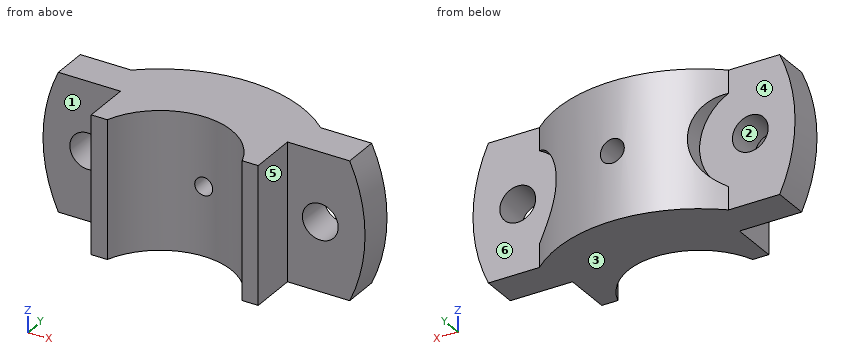
```python
from build123d import *

# Parameters (mm, degrees)
BOSS_EXTRUDE1_DEPTH     = 23
BOSS_EXTRUDE4_START     = 24
BOSS_EXTRUDE4_DEPTH     = 12
SKETCH4_R               = 3
CUT_EXTRUDE1_DEPTH      = 13
CUT_EXTRUDE1_DEPTH_BACK = 29
SKETCH5_R               = 4
CUT_EXTRUDE2_DEPTH      = 16
F_12_0MM_DOWEL_HOLE1_D  = 12
CUT_EXTRUDE3_DEPTH      = 16


with BuildPart() as part:
    # Sketch1 → Boss-Extrude1 (new body, symmetric)
    with BuildSketch(Plane.XY):
        with BuildLine():
            Line((31.749015733, 36), (31.749015733, 24))
            Line((31.749015733, 24), (28, 24))
            Line((28, 24), (28, 8))
            Line((28, 8), (22.627416998, 8))
            ThreePointArc((22.627416998, 8), (0, 24), (-22.627416998, 8))
            Line((-22.627416998, 8), (-28, 8))
            Line((-28, 8), (-28, 24))
            Line((-28, 24), (-31.749015733, 24))
            Line((-31.749015733, 24), (-31.749015733, 36))
            ThreePointArc((-31.749015733, 36), (0, 48), (31.749015733, 36))
        make_face()
    extrude(amount=BOSS_EXTRUDE1_DEPTH, both=True)

    # Sketch3 → Boss-Extrude4 (add)
    with BuildSketch(Plane(origin=(0, 0, 0), x_dir=(1, 0, 0), z_dir=(0, 1, 0)).offset(BOSS_EXTRUDE4_START)):
        with BuildLine():
            Line((31.749015733, -23), (31.749015733, 23))
            Line((31.749015733, 23), (48.856934001, 23))
            ThreePointArc((48.856934001, 23), (54, 0), (48.856934001, -23))
            Line((48.856934001, -23), (31.749015733, -23))
        make_face()
    boss_extrude4 = extrude(amount=BOSS_EXTRUDE4_DEPTH)

    # Mirror2: Boss-Extrude4 across plane
    add(boss_extrude4.mirror(Plane(origin=(0, 0, 0), x_dir=(0, 0, 1), z_dir=(1, 0, 0))))

    # Sketch4 → Cut-Extrude1 (cut, two sides)
    with BuildSketch(Plane(origin=(0, 36, 0), x_dir=(1, 0, 0), z_dir=(0, 1, 0))) as cut_extrude1_sk:
        Circle(SKETCH4_R)
    extrude(amount=CUT_EXTRUDE1_DEPTH, mode=Mode.SUBTRACT)
    extrude(cut_extrude1_sk.sketch, amount=-CUT_EXTRUDE1_DEPTH_BACK, mode=Mode.SUBTRACT)

    # Sketch5 → Cut-Extrude2 (cut)
    with BuildSketch(Plane(origin=(0, 48, 0), x_dir=(1, 0, 0), z_dir=(0, 1, 0))):
        Circle(SKETCH5_R)
    extrude(amount=-CUT_EXTRUDE2_DEPTH, mode=Mode.SUBTRACT)

    # Ø12.0mm Dowel Hole1 (through all)
    with Locations(Plane(origin=(0, 36, 0), x_dir=(1, 0, 0), z_dir=(0, 1, 0))):
        with Locations((-39, 0), (39, 0)):
            Hole(F_12_0MM_DOWEL_HOLE1_D / 2)

    # Sketch8 → Cut-Extrude3 (cut)
    with BuildSketch(Plane(origin=(0, 36, 0), x_dir=(1, 0, 0), z_dir=(0, 1, 0))):
        with BuildLine():
            Line((31.749015733, -15.376060196), (31.749015733, 15.376060196))
            ThreePointArc((31.749015733, 15.376060196), (22, 0), (31.749015733, -15.376060196))
        make_face()
    cut_extrude3 = extrude(amount=CUT_EXTRUDE3_DEPTH, mode=Mode.SUBTRACT)

    # Mirror3: Cut-Extrude3 across plane
    add(cut_extrude3.mirror(Plane(origin=(0, 0, 0), x_dir=(0, 0, 1), z_dir=(1, 0, 0))), mode=Mode.SUBTRACT)


solid = part.part
```
Work out the finished part from the listing and answer in its coordinate system (mm). Face numbers are marked on the shaded views. A direction names the side the tool comes from. Coordinates: 2 decimals unless noted, no trailing zeros. Order: outer loops, then holes, each group sorted by start corner. A loop starts at its lowest first (then second) coordinate and runs counter-clockwise, first axis right, second up. Notation, with made-up numbers: (49, 8.25) - (80, 8.25) arc R30 ccw to (80, 39.25) - close; hole circle Ø8 at (7.5, 13.5). An arc over 180 degrees is marked (long way). Answer as a JSON object with one key per item and string values.
1. The mould has two halves that part along Z. Classify the marked faces 1, 2 and 3: +Z half, -Z half, draft (parallel to the pull), parting line (faces both ways), or undercut.
Output values:
{"face 1": "draft", "face 2": "undercut", "face 3": "-Z half"}
2. Find section A-A on x = 39. Determine the outline of the cut face in (y, z), plus the area to 3 significant figures.
Output values:
{"outline": "(24, -23) - (36, -23) - (36, -6) - (24, -6) - close; (24, 6) - (36, 6) - (36, 23) - (24, 23) - close", "area": "408 mm²"}
3. Find section D-D on y = 20.5. Determine the outline of the cut face in (x, z), plus the area to 3 significant figures.
Output values:
{"outline": "(-28, -23) - (-12.48, -23) - (-12.48, 23) - (-28, 23) - close; (12.48, -23) - (28, -23) - (28, 23) - (12.48, 23) - close", "area": "1,430 mm²"}
4. Find section B-B on y = 28.5. Determine the outline of the cut face in (x, z).
Output values:
{"outline": "(-48.86, -23) - (48.86, -23) arc R54 ccw to (48.86, 23) - (-48.86, 23) arc R54 ccw to start; hole circle Ø12 at (-39, 0); hole circle Ø6 at (0, 0); hole circle Ø12 at (39, 0)"}
5. A tool of negligible diameter and unlimited length cuts with its end or side. For the marked faces 4, 5 and 6, from which of +Z, -Z, +X, -X, +Y, -Y can it reach the whole face along a straight path? Write none if from no direction.
Output values:
{"face 4": "-X, +Y", "face 5": "+Z, -Z, +X, -Y", "face 6": "+X, +Y"}
6. Consider line 1 (Z direction, x = -39, y = 31.5); line 2 (X direction, y = 37.5, z = 0); line 3 (Z direction, x = 0, y = 45). Determine where each line is inside the solid, lowest interval first.
Output values:
{"line 1": "z = -23 to -6, 6 to 23", "line 2": "x = -22 to -4, 4 to 22", "line 3": "z = -23 to -4, 4 to 23"}
7. Each of these flat-tipped pins is pushed along its axis until it touches: P1, Ø13, axis at x = 0, z = 0, coming from the -Y side; P2, Ø9.5, axis at x = 42.5, z = -10.5, coming from the +Y side; P3, Ø5, axis at y = 17.5, z = 1.5, coming from the +X side. Where does it stop, or does it pass through?
Output values:
{"P1": "stops at y = 23.1", "P2": "stops at y = 36", "P3": "stops at x = 28"}
8. Find section C-C on z = 0. Count the separate pieces of the cut face and the enclosed holes in it, plus the area to 3 significant figures.
Output values:
{"separate pieces": "4", "enclosed holes": "0", "area": "1,650 mm²"}
